from build123d import *

# Parameters (mm, degrees)
F0_R     = 3
F1_DEPTH = 3


with BuildPart() as f1:
    # F0 (on Front) → F1 (new body)
    with BuildSketch(Plane.XZ):
        with BuildLine():
            Line((10, 0), (10, 11))
            ThreePointArc((10, 11), (0, 1), (-10, 11))
            Line((-10, 11), (-10, 0))
            Line((-10, 0), (10, 0))
        make_face()
        with BuildLine():
            ThreePointArc((-10, 11), (0, 1), (10, 11))
            ThreePointArc((10, 11), (0, 21), (-10, 11))
        make_face()
        with Locations((0, 11)):
            Circle(F0_R, mode=Mode.SUBTRACT)
    extrude(amount=F1_DEPTH)

    # F2: F1 across face


with BuildPart() as f1_1:
    add(f1.part)
    add(f1.part.mirror(Plane(origin=(0, -1.5, 0), x_dir=(1, 0, 0), z_dir=(0, 0, -1))))


solid = f1_1.part
CAD build for the part. Positions are in the model's coordinates, mm. Round coordinates to 2 decimals unless told otherwise and drop trailing zeros. Write each loop counter-clockwise with the first axis right and the second up, starting at its lowest first coordinate (ties: lowest second). Pieces come first, ordered by that corner, then holes. Notation, with made-up numbers: (67, -21) -> (109, -21) arc R10 ccw to (109, -3) -> close; hole circle Ø1 at (10.5, 57). An arc over 180 degrees is marked (long way). Answer as a JSON object with one key per item and string values.
(1) Pin check, flat tip, straight feed: P1, Ø8, axis at x = -2.5, z = 13.5, coming from the +Y side. Stop position of the tip, or through.
Reported:
{"P1": "stops at y = 0"}
(2) Two-plate mould, pull along Z, no slides. Class faces 1 (the face through (0, -1, -21)), 2 (the face through (-0.65, -1.48, -8.07)), 3 (the face through (-0.65, -1.48, 8.07)), 4 (the face through (10, -1, 0)): +Z half, -Z half, draft (parallel to the pull), parting line (faces both ways), or undercut.
Reported:
{"face 1": "-Z half", "face 2": "undercut", "face 3": "undercut", "face 4": "draft"}
(3) Band-saw the part on D-D, the plane z = 14.5. List the corners of the cut face in (x, y).
Reported:
{"outline": "(-9.37, -3) -> (9.37, -3) -> (9.37, 0) -> (-9.37, 0) -> close"}
(4) Band-saw the part on A-A, the plane x = 0. List the corners of the cut face in (y, z), then the cut area to 3 significant figures.
Reported:
{"outline": "(-3, -21) -> (0, -21) -> (0, -14) -> (-3, -14) -> close; (-3, -8) -> (0, -8) -> (0, 8) -> (-3, 8) -> close; (-3, 14) -> (0, 14) -> (0, 21) -> (-3, 21) -> close", "area": "90.0 mm^2"}
(5) Probe probe 1 along Z at (x, y) = (0, -1.7); probe 2 along Z at (x, y) = (-1, -1.25); probe 3 along X at (y, z) = (-1.6, -11). List the from-to ranges inside material, lowest first. Write a range as [from, to].
Reported:
{"probe 1": "z = [-21, -14], [-8, 8], [14, 21]", "probe 2": "z = [-20.95, -13.83], [-8.17, 8.17], [13.83, 20.95]", "probe 3": "x = [-10, -3], [3, 10]"}
(6) Band-saw the part on C-C, the plane x = -8. List the corners of the cut face in (y, z).
Reported:
{"outline": "(-3, -17) -> (0, -17) -> (0, 17) -> (-3, 17) -> close"}
(7) Band-saw the part on B-B, the plane y = -2.05. List the corners of the cut face in (x, z), then the cut area to 3 significant figures.
Reported:
{"outline": "(-10, -11) arc R10 ccw to (10, -11) -> (10, 11) arc R10 ccw to (-10, 11) -> close; hole circle Ø6 at (0, -11); hole circle Ø6 at (0, 11)", "area": "698 mm^2"}
